Can you work these out from the drawing? Everything is in mm from the part's minimum corner. A direction names the side the tool comes from. Round coordinates to 2 decimals unless told otherwise and drop trailing zeros. Order: outer loops, then holes, each group sorted by start corner. A loop starts at its lowest first (then second) coordinate and runs counter-clockwise, first axis right, second up. Notation, with made-up numbers: M -0.75,-35 L 28.25,-35 A28 ccw 28.25,-13 Z; hole C -2,-27.5 d1. An arc over 180 degrees is marked long. Answer as a JSON object with one key per item and string values. Group by question number.
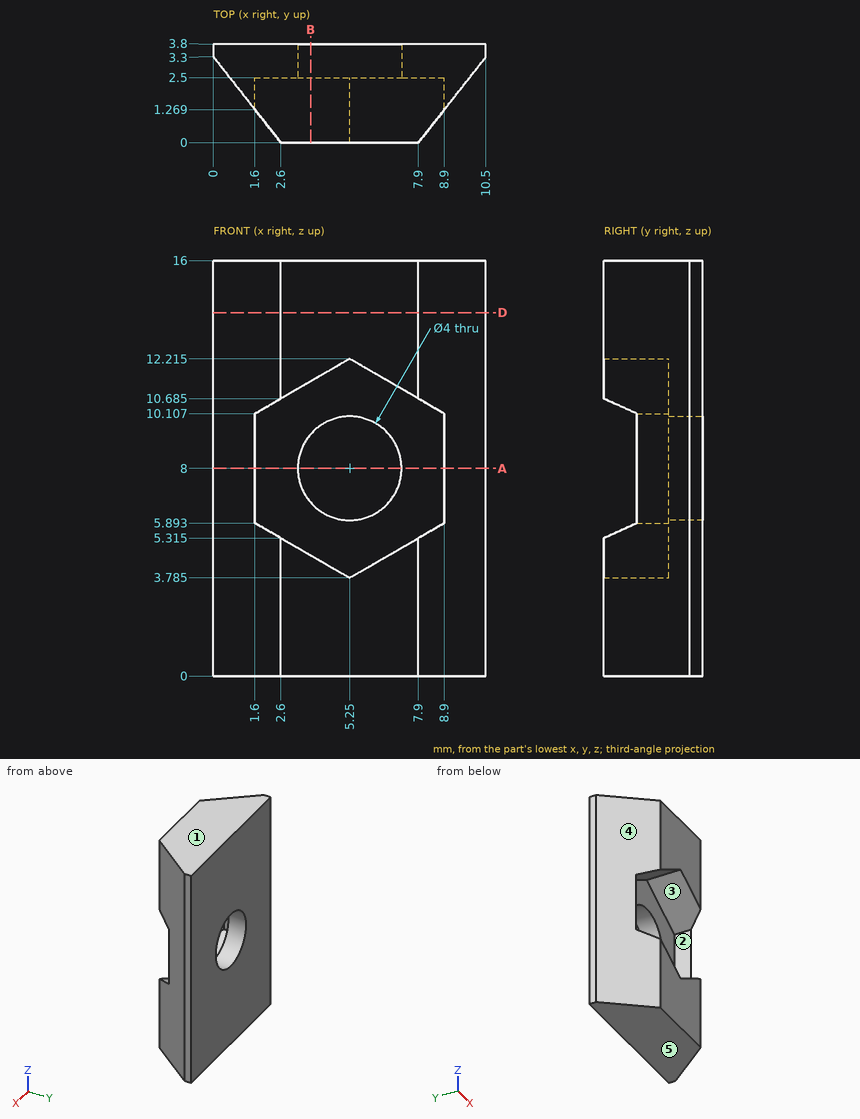
Item 1: Suppose I cut it at D-D, the plane z = 14. Write out the boundary of the cut face in (x, y).
Item 2: Suppose I cut it at B-B, the plane x = 3.75. Write out the boundary of the cut face in (y, z).
Item 3: On a 3-axis mill with a long thin cutter (end or side, diameter ignored), from which of +Z, -Z, +X, -X, +Y, -Y can I reach the whole of each face in a straight line? I mean the marked faces 1 and 2. Say none if no direction works.
Item 4: If we mould it in two halves opening along X, with no side actions, what happens to the marked faces 3, 4 and 5? For each: +X half, -X half, draft (parallel to the pull), parting line (faces both ways), or undercut.
Item 5: I need wall thicknesses on line 1 (X direction, y = 3.55, z = 8); line 2 (Z direction, x = 5.25, y = 2.8); line 3 (X direction, y = 3.15, z = 8). Which ranges of each line are inside material? Lowest first, please.
Item 6: Suppose I cut it at A-A, the plane z = 8. Write out the boundary of the cut face in (x, y).
Item 7: I'm going to push flat-ended pins straight in: pin 1 Ø1.4 at (y, z) = (2, 8.5) entering from -X; pin 2 Ø0.6 at (y, z) = (2, 9) entering from +X. Where does each tip first touch, or does it pass through?
Computed:
{
 "1": {"outline": "M 0,3.3 L 2.6,0 L 7.9,0 L 10.5,3.3 L 10.5,3.8 L 0,3.8 Z"},
 "2": {"outline": "M 0,0 L 3.8,0 L 3.8,6.68 L 2.5,6.68 L 2.5,4.65 L 0,4.65 Z; M 0,11.35 L 2.5,11.35 L 2.5,9.32 L 3.8,9.32 L 3.8,16 L 0,16 Z"},
 "3": {"face 1": "+Z, +X, -X, +Y, -Y", "face 2": "-Y"},
 "4": {"face 3": "undercut", "face 4": "-X half", "face 5": "draft"},
 "5": {"line 1": "x = 0 to 3.25, 7.25 to 10.5", "line 2": "z = 0 to 6, 10 to 16", "line 3": "x = 0.12 to 3.25, 7.25 to 10.38"},
 "6": {"outline": "M 0,3.3 L 1.6,1.27 L 1.6,2.5 L 3.25,2.5 L 3.25,3.8 L 0,3.8 Z; M 7.25,2.5 L 8.9,2.5 L 8.9,1.27 L 10.5,3.3 L 10.5,3.8 L 7.25,3.8 Z"},
 "7": {"pin 1": "stops at x = 0.47", "pin 2": "stops at x = 9.71"}
}
